Geometry: final body of the model. Coordinates: model frame, mm. A direction names the side the tool comes from. Coordinates: 2 decimals unless noted, no trailing zeros. Write each loop counter-clockwise with the first axis right and the second up, starting at its lowest first coordinate (ties: lowest second). Pieces come first, ordered by that corner, then holes. Notation, with made-up numbers: (22, 53) - (32, 53) arc R13 ccw to (32, 64) - close; hole circle Ø7 at (17, 38). An arc over 180 degrees is marked (long way). Put each result on its own line as item: value.
```python
from build123d import *

# Parameters (mm, degrees)
SKETCH1_W           = 82.2198
SKETCH1_H           = 54.2544
BOSS_EXTRUDE1_DEPTH = 9.525
SKETCH2_W           = 82.2198
SKETCH2_H           = 4.4831
BOSS_EXTRUDE2_DEPTH = 1.3589
SKETCH3_W           = 54.2544
SKETCH3_H           = 4.4831
BOSS_EXTRUDE3_DEPTH = 1.3589


with BuildPart() as part:
    # Sketch1 → Boss-Extrude1 (new body)
    with BuildSketch(Plane(origin=(0, 0, 0), x_dir=(1, 0, 0), z_dir=(0, 1, 0))):
        Rectangle(SKETCH1_W, SKETCH1_H)
    extrude(amount=BOSS_EXTRUDE1_DEPTH)

    # Sketch2 → Boss-Extrude2 (add)
    with BuildSketch(Plane.XY.offset(27.1272)):
        with Locations((0, 2.24155)):
            Rectangle(SKETCH2_W, SKETCH2_H)
    boss_extrude2 = extrude(amount=BOSS_EXTRUDE2_DEPTH)

    # Mirror1: Boss-Extrude2 across plane
    add(boss_extrude2.mirror(Plane.XY))

    # Sketch3 → Boss-Extrude3 (add)
    with BuildSketch(Plane(origin=(41.1099, 0, 0), x_dir=(0, 0, -1), z_dir=(1, 0, 0))):
        with Locations((0, 2.24155)):
            Rectangle(SKETCH3_W, SKETCH3_H)
    boss_extrude3 = extrude(amount=BOSS_EXTRUDE3_DEPTH)

    # Mirror2: Boss-Extrude3 across plane
    add(boss_extrude3.mirror(Plane(origin=(0, 0, 0), x_dir=(0, 0, 1), z_dir=(1, 0, 0))))


solid = part.part
```
1. Section query C-C (y = 6.25). Return loops of the section in (x, z), then the cut area to 3 significant figures.
Answer below:
outline: (-41.11, -27.13) - (41.11, -27.13) - (41.11, 27.13) - (-41.11, 27.13) - close
area: 4,460 mm²
2. Section query B-B (x = 37.5). Return loops of the section in (y, z) (3 decimals).
Answer below:
outline: (0, -28.486) - (4.483, -28.486) - (4.483, -27.127) - (9.525, -27.127) - (9.525, 27.127) - (4.483, 27.127) - (4.483, 28.486) - (0, 28.486) - close
3. Ray query, probe 1 along Z at (x, y) = (9, 6.75); probe 2 along X at (y, z) = (5, 6). Return the intervals inside material, ascending. Write a range as from..to.
Answer below:
probe 1: z = -27.13..27.13
probe 2: x = -41.11..41.11
4. Pin query (flat end, axial travel): pin 1 Ø0.7 at (x, z) = (-19, -28) entering from +Y; pin 2 Ø4 at (x, y) = (9, 7.5) entering from -Z; pin 3 Ø5.5 at (y, z) = (7.5, 9) entering from -X. Return the tip coordinate at first contact, or that it passes through.
Answer below:
pin 1: stops at y = 4.48
pin 2: stops at z = -27.13
pin 3: stops at x = -41.11
5. Set-up query: faces 1 (the flat face through (41.11, 7, 0)), 2 (the flat face through (42.469, 2, 0)), 3 (the flat face through (-1, 7, -27.127)), 4 (the flat face through (-1, 7, 27.127)), 5 (the flat face through (-41.11, 7, 0)). Return all of +Z, -Z, +X, -X, +Y, -Y with unobstructed straight access to the full face (end or side cutting, diameter ignored); none if empty.
Answer below:
face 1: +Z, -Z, +X, +Y
face 2: +Z, -Z, +X, +Y, -Y
face 3: -Z, +X, -X, +Y
face 4: +Z, +X, -X, +Y
face 5: +Z, -Z, -X, +Y
6. Section query A-A (z = 11). Return loops of the section in (x, y) (3 decimals).
Answer below:
outline: (-42.469, 0) - (42.469, 0) - (42.469, 4.483) - (41.11, 4.483) - (41.11, 9.525) - (-41.11, 9.525) - (-41.11, 4.483) - (-42.469, 4.483) - close
